The model under review builds one solid part; all positions refer to its coordinate system, in mm. Face numbers are marked on the shaded views. A direction names the side the tool comes from. Coordinates: 2 decimals unless noted, no trailing zeros. Loops run counter-clockwise (first coordinate to the right, second up) from the corner with the lowest first, then second, coordinate; pieces in that order, holes last. Notation, with made-up numbers: M 30,75 L 44,75 A19 ccw 44,103 Z; hole C 51,31 d3. An arc over 180 degrees is marked long. Return JSON: item names as keys, results as strings.
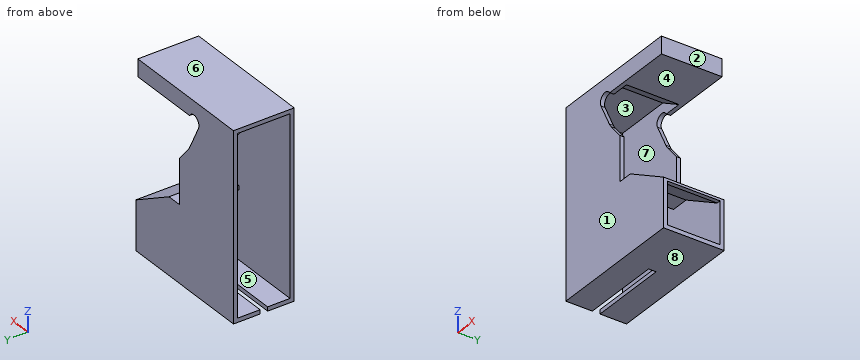
```python
from build123d import *

# Parameters (mm, degrees)
F0_R         = 2.3
F1_DEPTH     = 8.8
F2_T         = -1.2
F3_DEPTH     = 1.2
F4_DEPTH     = 28.2
F5_DEPTH     = 1.2
F6_W         = 23
F6_H         = 2.2
F7_DEPTH     = 1.2
F9_DEPTH     = 17.6
F10_W        = 15.2
F10_H        = 3.8
F11_DEPTH    = 25
F12_T4_DEPTH = 15.2


# Not quite as in the source:
# - a fillet or chamfer that OpenCascade refuses, or shapes differently, is made with other operations: its cross-section is extruded or revolved along the edge and cut away or added
# - a feature names something its author has since deleted; it is built from what else it names


with BuildPart() as f1:
    # F0 (on Front) → F1 (new body, symmetric)
    with BuildSketch(Plane.XZ):
        Polygon((-40.0227420032, 54), (-40.0227420032, 0), (0, 0), (0, 14.1528282114), (-13.5917002335, 22), (-17.8529980872, 22), (-17.8529980872, 49), (-0.8529980872, 49), (-0.8529980872, 54), (-17.8529980872, 54), align=None)
        with Locations((-24.1529980872, 48.7)):
            Circle(F0_R, mode=Mode.SUBTRACT)
        with Locations((-24.1529980872, 48.7)):
            Circle(F0_R)
    extrude(amount=F1_DEPTH, both=True)

    # F2
    f2_openings = [f1.faces().sort_by_distance(p)[0] for p in [
        (-40.022742, 0, 27),
    ]]
    offset(amount=F2_T, openings=f2_openings, kind=Kind.INTERSECTION)

    # F3 (cut, through all): a face of the model
    f3_faces = [f1.faces().sort_by_distance(p)[0] for p in [
        (-2.0529980872, 0, 51.5),
    ]]
    extrude(f3_faces, amount=-F3_DEPTH, mode=Mode.SUBTRACT)

    # F4 (cut, through all): a face of the model
    f4_faces = [f1.faces().sort_by_distance(p)[0] for p in [
        (-9.9529980872, 0, 50.2),
    ]]
    extrude(f4_faces, amount=-F4_DEPTH, mode=Mode.SUBTRACT)

    # F5 (cut, through all): a face of the model
    f5_faces = [f1.faces().sort_by_distance(p)[0] for p in [
        (-1.2, 0, 7.3300039442),
    ]]
    extrude(f5_faces, amount=-F5_DEPTH, mode=Mode.SUBTRACT)

    # F6 (on face) → F7 (cut, through all)
    with BuildSketch(Plane(origin=(0, 0, 0), x_dir=(1, 0, 0), z_dir=(0, 0, -1))):
        with Locations((-28.5227420032, 0)):
            Rectangle(F6_W, F6_H)
    extrude(amount=-F7_DEPTH, mode=Mode.SUBTRACT)

    # F8 (on face) → F9 (cut, through all)
    with BuildSketch(Plane.XZ.offset(8.8)):
        with BuildLine():
            ThreePointArc((-22.2107439409, 40.3830760217), (-22.207256, 45.7916724587), (-17.8529980872, 49))
            Line((-17.8529980872, 49), (-21.9990858511, 49))
            Line((-21.9990858511, 49), (-22.3439980513, 49.3965202671))
            ThreePointArc((-22.3439980513, 49.3965202671), (-24.9680683048, 49.7442269385), (-25.6389133718, 47.1836388185))
            Line((-25.6389133718, 47.1836388185), (-22.2107439409, 40.3830760217))
        make_face()
        with BuildLine():
            Line((-17.8529980872, 34.9413308483), (-17.8529980872, 49))
            ThreePointArc((-17.8529980872, 49), (-22.207256, 45.7916724587), (-22.2107439409, 40.3830760217))
            ThreePointArc((-22.2107439409, 40.3830760217), (-21.8634478438, 39.783103161), (-21.4492647459, 39.2271945588))
            Line((-21.4492647459, 39.2271945588), (-17.8529980872, 34.9413308483))
        make_face()
    extrude(amount=-F9_DEPTH, mode=Mode.SUBTRACT)

    # F10 (on face) → F11 (join)
    with BuildSketch(Plane.YZ.offset(-0.8529980872)):
        with Locations((0, 50.9)):
            Rectangle(F10_W, F10_H)
    extrude(amount=-F11_DEPTH)

    # F12: chamfer of 9 x 5.1961524227 on 1 edges, made by hand


with BuildPart() as f12_tool2:
    # F12_s3 → F12_t4 (new body)
    with BuildSketch(Plane.XZ.offset(7.6)):
        Polygon((-16.8529980872, 49), (-25.8529980872, 54.1961524227), (-25.8529980872, 49), align=None)
    extrude(amount=-F12_T4_DEPTH)

    split(bisect_by=Plane.XY.offset(52.8), keep=Keep.BOTTOM)


with BuildPart() as f1_1:
    add(f1.part)

    # F12_t1: cut F12_tool2
    add(f12_tool2.part, mode=Mode.SUBTRACT)


solid = f1_1.part
```
1. Add section B-B on z = 7. Give the boundary of the cut face in (x, y), plus the area to 3 significant figures.
Check values:
{"outline": "M -40.02,-8.8 L 0,-8.8 L 0,-7.6 L -40.02,-7.6 Z; M -40.02,7.6 L 0,7.6 L 0,8.8 L -40.02,8.8 Z", "area": "96.1 mm²"}
2. Add section D-D on x = -20.5. Give the boundary of the cut face in (y, z).
Check values:
{"outline": "M -8.8,0 L -1.1,0 L -1.1,1.2 L -7.6,1.2 L -7.6,38.1 L -8.8,38.1 Z; M -8.8,49 L -7.6,49 L -7.6,51.11 L 7.6,51.11 L 7.6,49 L 8.8,49 L 8.8,54 L -8.8,54 Z; M 1.1,0 L 8.8,0 L 8.8,38.1 L 7.6,38.1 L 7.6,1.2 L 1.1,1.2 Z"}
3. Machinability: for the marked faces 1, 2, 3, 4 and 5, which of the approach directions +Z, -Z, +X, -X, +Y, -Y give a long, thin tool a straight path to every point of the face, cutting with its end or side? Answer none if there is none.
Check values:
{"face 1": "+Z, -Z, +X, -X, -Y", "face 2": "+Z, +X, +Y, -Y", "face 3": "-X", "face 4": "+X, +Y, -Y", "face 5": "+X, -X"}
4. The part is to be moulded in two halves that separate along Z. For the marked faces 6, 7 and 8, say which applies: released by +Z, released by -Z, zero draft, split by the parting line, or undercut.
Check values:
{"face 6": "released by +Z", "face 7": "undercut", "face 8": "released by -Z"}
5. To check wall thickness, follow line 1 (Z direction, x = -34.5, y = 4); line 2 (Y direction, x = -28.5, z = 47); line 3 (Z direction, x = -3.5, y = -6.25). State the ranges of each line that lie inside material, in increasing order.
Check values:
{"line 1": "0 to 1.2, 52.8 to 54", "line 2": "-8.8 to -7.6, 7.6 to 8.8", "line 3": "0 to 1.2, 14.79 to 16.17, 49 to 54"}
6. Add section A-A on x = -15.5. Give the boundary of the cut face in (y, z).
Check values:
{"outline": "M -8.8,0 L 8.8,0 L 8.8,22 L -8.8,22 Z; M -8.8,49 L 8.8,49 L 8.8,54 L -8.8,54 Z; hole M -7.6,1.2 L 7.6,1.2 L 7.6,20.8 L -7.6,20.8 Z"}
7. Insertion check: pin 1 Ø1.5 at (x, y) = (-17.5, -2.5) entering from -Z; pin 2 Ø0.6 at (y, z) = (0, 0.5) entering from -X; pin 3 Ø1 at (y, z) = (8, 29.5) entering from +X; pin 4 Ø1.5 at (y, z) = (-3, 51.5) entering from +X. Each pin has a flat end and moves straight along its axis. Give the tip position at first contact, or say it passes through.
Check values:
{"pin 1": "z = 0", "pin 2": "x = -17.02", "pin 3": "x = -17.85", "pin 4": "x = -0.85"}
8. Add section C-C on y = 0. Give the boundary of the cut face in (x, z), plus the area to 3 significant figures.
Check values:
{"outline": "M -40.02,52.8 L -23.43,52.8 L -16.85,49 L -0.85,49 L -0.85,54 L -40.02,54 Z; M -19.05,20.8 L -13.91,20.8 L -1.2,13.46 L 0,13.46 L 0,14.15 L -13.59,22 L -19.05,22 Z; M -17.02,0 L 0,0 L 0,1.2 L -17.02,1.2 Z", "area": "166 mm²"}
